```python
from build123d import *

# Parameters (mm, degrees)
PAD_DEPTH       = 25
SKETCH001_W     = 91
SKETCH001_H     = 26
POCKET_DEPTH    = 25.001
SKETCH002_R     = 1.5
POCKET001_DEPTH = 3
SKETCH004_R     = 1
POCKET002_DEPTH = 5
SKETCH005_R     = 8.5
SKETCH005_R_2   = 2.5
SKETCH005_R_3   = 2.25
SKETCH005_R_4   = 0.5
POCKET003_DEPTH = 0.5
SKETCH006_R     = 1.5
POCKET004_DEPTH = 5


with BuildPart() as part:
    # Sketch → Pad (new body)
    with BuildSketch(Plane.XZ):
        with BuildLine():
            ThreePointArc((-32.5, 12.5), (-45, 0), (-32.5, -12.5))
            Line((-32.5, -12.5), (32.5, -12.5))
            ThreePointArc((32.5, -12.5), (45, 0), (32.5, 12.5))
            Line((-32.5, 12.5), (32.5, 12.5))
        make_face()
    extrude(amount=-PAD_DEPTH)

    # Sketch001 (on Face4 of Pad) → Pocket (cut, through all)
    with BuildSketch(Plane(origin=(0, 0, 12.5), x_dir=(-1, 0, 0), z_dir=(0, 0, 1))):
        with Locations((0, -12.5)):
            Rectangle(SKETCH001_W, SKETCH001_H)
        Polygon((45, -16), (45, -2), (45, 0), (44, 0), (-32.5, 0), (-44.5, 0), (-45, 0), (-45, -3.68), (-45, -23), (-45, -25), (-44, -25), (40, -25), (40, -16), align=None, mode=Mode.SUBTRACT)
    extrude(amount=-POCKET_DEPTH, mode=Mode.SUBTRACT)

    # Sketch002 (on Face5 of Pocket) → Pocket001 (cut)
    with BuildSketch(Plane(origin=(0, 25, 0), x_dir=(1, 0, 0), z_dir=(0, 1, 0))):
        with Locations((22.5, 0)):
            Circle(SKETCH002_R)
        with Locations((-22.5, 0)):
            Circle(SKETCH002_R)
    extrude(amount=-POCKET001_DEPTH, mode=Mode.SUBTRACT)

    # Sketch004 (on Face7 of Pocket001) → Pocket002 (cut)
    with BuildSketch(Plane(origin=(-40, 0, 0), x_dir=(0, 0, -1), z_dir=(-1, 0, 0))):
        with Locations((-7.5, -20.28)):
            Circle(SKETCH004_R)
        with Locations((7.5, -20.28)):
            Circle(SKETCH004_R)
        with BuildLine():
            ThreePointArc((-3.3, -19.08), (-4.5, -20.28), (-3.3, -21.48))
            Line((-3.3, -21.48), (3.3, -21.48))
            ThreePointArc((3.3, -21.48), (4.5, -20.28), (3.3, -19.08))
            Line((-3.3, -19.08), (3.3, -19.08))
        make_face()
    extrude(amount=-POCKET002_DEPTH, mode=Mode.SUBTRACT)

    # Sketch005 (on Face1 of Pocket002) → Pocket003 (cut)
    with BuildSketch(Plane.XZ):
        with Locations((-22.5, 0)):
            Circle(SKETCH005_R)
        with Locations((-22.5, 0)):
            Circle(SKETCH005_R_2, mode=Mode.SUBTRACT)
        with Locations((22.5, 0)):
            Circle(SKETCH005_R)
        with Locations((22.5, 0)):
            Circle(SKETCH005_R_2, mode=Mode.SUBTRACT)
        Circle(SKETCH005_R_3)
        Circle(SKETCH005_R_4, mode=Mode.SUBTRACT)
    extrude(amount=-POCKET003_DEPTH, mode=Mode.SUBTRACT)

    # Sketch006 (on Face5 of Pocket003) → Pocket004 (cut)
    with BuildSketch(Plane(origin=(0, 0, -12.5), x_dir=(1, 0, 0), z_dir=(0, 0, -1))):
        with Locations((-17, -12.5)):
            Circle(SKETCH006_R)
        with Locations((17, -12.5)):
            Circle(SKETCH006_R)
    extrude(amount=-POCKET004_DEPTH, mode=Mode.SUBTRACT)


solid = part.part
```
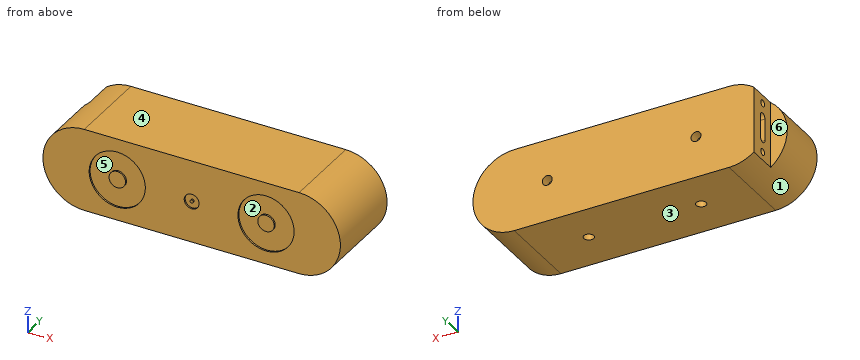
The model under review builds one solid part; all positions refer to its coordinate system, in mm. Face numbers are marked on the shaded views. A direction names the side the tool comes from. Give positions to 0.01 mm unless a question says otherwise; leave off trailing zeros. Loops run counter-clockwise (first coordinate to the right, second up) from the corner with the lowest first, then second, coordinate; pieces in that order, holes last. Notation, with made-up numbers: (65.25, 2) -> (120.25, 2) arc R11 ccw to (120.25, 10) -> close; hole circle Ø7 at (80.5, 56.25). An arc over 180 degrees is marked (long way). Use CSV: the item, a comma, the result in double quotes.
1. To check wall thickness, follow probe 1 along Z at (x, y) = (-22.5, 0.2); probe 2 along Y at (x, z) = (-37.25, -7.5); probe 3 along Z at (x, y) = (22.5, 22.75). State the ranges of each line that lie inside material, in increasing order. Write a range as from..to.
Result:
probe 1,"z = -12.5..-8.5, -2.5..2.5, 8.5..12.5"
probe 2,"y = 0..19.28, 21.28..25"
probe 3,"z = -12.5..-1.5, 1.5..12.5"
2. For P1, Ø12, axis at y = 19, z = -8.5, coming from the -X side; P2, Ø0.9, axis at x = -17, y = 12, coming from the -Z side; P3, Ø1.5, axis at x = -22, z = 0.5, coming from the +Y side, all flat-tipped, find the tip position at first contact; note any pin that passes through.
Result:
P1,"stops at x = -44.56"
P2,"stops at z = -7.5"
P3,"stops at y = 22"
3. Consider section D-D, the plane y = 20.28. Write out the cut boundary in (x, z).
Result:
outline,"(-40, -10) arc R12.5 ccw to (-32.5, -12.5) -> (32.5, -12.5) arc R12.5 ccw to (32.5, 12.5) -> (-32.5, 12.5) arc R12.5 ccw to (-40, 10) -> (-40, 8.5) -> (-35, 8.5) -> (-35, 6.5) -> (-40, 6.5) -> (-40, 4.5) -> (-35, 4.5) -> (-35, -4.5) -> (-40, -4.5) -> (-40, -6.5) -> (-35, -6.5) -> (-35, -8.5) -> (-40, -8.5) -> close"
4. Consider section A-A, the plane z = 7.5. Write out the cut boundary in (x, y), then the cut area to 3 significant figures.
Result:
outline,"(-42.5, 0) -> (-26.5, 0) -> (-26.5, 0.5) -> (-18.5, 0.5) -> (-18.5, 0) -> (18.5, 0) -> (18.5, 0.5) -> (26.5, 0.5) -> (26.5, 0) -> (42.5, 0) -> (42.5, 25) -> (-40, 25) -> (-40, 21.28) -> (-35, 21.28) -> (-35, 19.28) -> (-40, 19.28) -> (-40, 16) -> (-42.5, 16) -> close"
area,"2,080 mm²"
5. The part is to be moulded in two halves that separate along X. For the marked faces 1, 2 and 3, say which applies: +X half, -X half, draft (parallel to the pull), parting line (faces both ways), or undercut.
Result:
face 1,"-X half"
face 2,"undercut"
face 3,"draft"
6. Consider section C-C, the plane x = 16.5. Write out the cut boundary in (y, z), then the cut area to 3 significant figures.
Result:
outline,"(0, -12.5) -> (11.09, -12.5) -> (11.09, -7.5) -> (13.91, -7.5) -> (13.91, -12.5) -> (25, -12.5) -> (25, 12.5) -> (0, 12.5) -> (0, 6.02) -> (0.5, 6.02) -> (0.5, -6.02) -> (0, -6.02) -> close"
area,"605 mm²"
7. Machinability: for the marked faces 4, 5 and 6, which of the approach directions +Z, -Z, +X, -X, +Y, -Y give a long, thin tool a straight path to every point of the face, cutting with its end or side? Answer none if there is none.
Result:
face 4,"+Z, +X, -X, +Y, -Y"
face 5,"-Y"
face 6,"+Z, -Z, -X, +Y"
8. Consider section B-B, the plane y = 12.5. Write out the cut boundary in (x, z).
Result:
outline,"(-32.5, -12.5) -> (-18.5, -12.5) -> (-18.5, -7.5) -> (-15.5, -7.5) -> (-15.5, -12.5) -> (15.5, -12.5) -> (15.5, -7.5) -> (18.5, -7.5) -> (18.5, -12.5) -> (32.5, -12.5) arc R12.5 ccw to (32.5, 12.5) -> (-32.5, 12.5) arc R12.5 ccw to start"
